from build123d import *

# Parameters (mm, degrees)
SKETCH_1_W          = 159
SKETCH_1_H          = 116
EXTRUDE_1_DEPTH     = 2
SKETCH_3_R          = 1.99
EXTRUDE_3_DEPTH     = 79.5
SKETCH_4_W          = 149
SKETCH_4_H          = 7
CUT_EXTRUDE_2_DEPTH = 79.5
FILLET_3_R          = 2


with BuildPart() as part:
    # 草图1 → 凸台-拉伸1 (new body)
    with BuildSketch(Plane(origin=(0, 0, 0), x_dir=(1, 0, 0), z_dir=(0, 1, 0))):
        Rectangle(SKETCH_1_W, SKETCH_1_H)
    extrude(amount=EXTRUDE_1_DEPTH)

    # 草图3 → 凸台-拉伸3 (add, symmetric)
    # profile 1 of 2: a face of its own
    with BuildSketch(Plane(origin=(0, 0, 0), x_dir=(0, 0, -1), z_dir=(1, 0, 0))):
        with BuildLine():
            Line((-57, 6), (-57, 2))
            Line((-57, 2), (-51, 2))
            Line((-51, 2), (-51, 6))
            ThreePointArc((-51, 6), (-54, 9), (-57, 6))
        make_face()
        with Locations(Location((-54, 6, 0), (0, 0, 180))):
            Circle(SKETCH_3_R, mode=Mode.SUBTRACT)
    # profile 2 of 2: a face of its own
    with BuildSketch(Plane(origin=(0, 0, 0), x_dir=(0, 0, -1), z_dir=(1, 0, 0))):
        with BuildLine():
            Line((51, 2), (51, 6))
            ThreePointArc((51, 6), (54, 9), (57, 6))
            Line((57, 6), (57, 2))
            Line((57, 2), (51, 2))
        make_face()
        with Locations(Location((54, 6, 0), (0, 0, 180))):
            Circle(SKETCH_3_R, mode=Mode.SUBTRACT)
    extrude(amount=EXTRUDE_3_DEPTH, both=True)

    # 草图4 → 切除-拉伸2 (cut, symmetric)
    with BuildSketch(Plane.XY):
        with Locations((0, 5.5)):
            Rectangle(SKETCH_4_W, SKETCH_4_H)
    extrude(amount=CUT_EXTRUDE_2_DEPTH, both=True, mode=Mode.SUBTRACT)

    # 圆角3
    # the kernel refuses this fillet: 2 mm, written as the material it adds along each edge
    with BuildSketch(Plane(origin=(74.5, 2, 57), x_dir=(0, 1, 0), z_dir=(1, 0, 0))) as fillet_3_piece_1:
        with BuildLine():
            CenterArc((1.732050808, 2), FILLET_3_R, 210, 60)
            Line((0, 1), (-0.034641016, 0.98))
            ThreePointArc((-0.034641016, 0.98), (-0.04, 0.5), (-0.04, 0))
            Line((-0.04, 0), (0, -0.04))
            Line((0, -0.04), (1.732050808, -0.04))
            Line((1.732050808, -0.04), (1.732050808, 0))
        make_face()
    extrude(amount=5)
    with BuildSketch(Plane(origin=(74.5, 2, 51), x_dir=(0, 1, 0), z_dir=(1, 0, 0)), Plane(origin=(-79.5, 2, -51), x_dir=(0, 0, 1), z_dir=(1, 0, 0))) as fillet_3_piece_2:
        with BuildLine():
            CenterArc((FILLET_3_R, -FILLET_3_R), FILLET_3_R, 90, 90)
            Line((0, -FILLET_3_R), (-FILLET_3_R * 0.02, -FILLET_3_R))
            Line((-FILLET_3_R * 0.02, -FILLET_3_R), (-FILLET_3_R * 0.02, FILLET_3_R * 0.02))
            Line((-FILLET_3_R * 0.02, FILLET_3_R * 0.02), (FILLET_3_R, FILLET_3_R * 0.02))
            Line((FILLET_3_R, FILLET_3_R * 0.02), (FILLET_3_R, 0))
        make_face()
    extrude(amount=5)
    with BuildSketch(Plane(origin=(74.5, 2, -51), x_dir=(0, 1, 0), z_dir=(1, 0, 0)), Plane(origin=(-79.5, 2, 51), x_dir=(0, 0, -1), z_dir=(1, 0, 0))) as fillet_3_piece_3:
        with BuildLine():
            CenterArc((FILLET_3_R, FILLET_3_R), FILLET_3_R, 180, 90)
            Line((0, FILLET_3_R), (-FILLET_3_R * 0.02, FILLET_3_R))
            Line((-FILLET_3_R * 0.02, FILLET_3_R), (-FILLET_3_R * 0.02, -FILLET_3_R * 0.02))
            Line((-FILLET_3_R * 0.02, -FILLET_3_R * 0.02), (FILLET_3_R, -FILLET_3_R * 0.02))
            Line((FILLET_3_R, -FILLET_3_R * 0.02), (FILLET_3_R, 0))
        make_face()
    extrude(amount=5)
    with BuildSketch(Plane(origin=(74.5, 2, -57), x_dir=(0, 1, 0), z_dir=(1, 0, 0))) as fillet_3_piece_4:
        with BuildLine():
            CenterArc((1.732050808, -2), FILLET_3_R, 90, 60)
            Line((0, -1), (-0.034641016, -0.98))
            ThreePointArc((-0.034641016, -0.98), (-0.04, -0.5), (-0.04, 0))
            Line((-0.04, 0), (0, 0.04))
            Line((0, 0.04), (1.732050808, 0.04))
            Line((1.732050808, 0.04), (1.732050808, 0))
        make_face()
    extrude(amount=5)
    with BuildSketch(Plane(origin=(-79.5, 2, -57), x_dir=(0, 0, -1), z_dir=(1, 0, 0))) as fillet_3_piece_5:
        with BuildLine():
            CenterArc((2, 1.732050808), FILLET_3_R, 180, 60)
            Line((0, 1.732050808), (-0.04, 1.732050808))
            Line((-0.04, 1.732050808), (-0.04, 0))
            Line((-0.04, 0), (0, -0.04))
            ThreePointArc((0, -0.04), (0.5, -0.04), (0.98, -0.034641016))
            Line((0.98, -0.034641016), (1, 0))
        make_face()
    extrude(amount=5)
    with BuildSketch(Plane(origin=(-79.5, 2, 57), x_dir=(0, 0, 1), z_dir=(1, 0, 0))) as fillet_3_piece_6:
        with BuildLine():
            CenterArc((2, -1.732050808), FILLET_3_R, 120, 60)
            Line((0, -1.732050808), (-0.04, -1.732050808))
            Line((-0.04, -1.732050808), (-0.04, 0))
            Line((-0.04, 0), (0, 0.04))
            ThreePointArc((0, 0.04), (0.5, 0.04), (0.98, 0.034641016))
            Line((0.98, 0.034641016), (1, 0))
        make_face()
    extrude(amount=5)


solid = part.part
Here's how the part is built. I have some questions about the finished solid (model axes, mm). A direction names the side the tool comes from. Coordinates: 2 decimals unless noted, no trailing zeros. Order: outer loops, then holes, each group sorted by start corner. A loop starts at its lowest first (then second) coordinate and runs counter-clockwise, first axis right, second up. Notation, with made-up numbers: M 15,-21.75 L 19,-21.75 A19 cw 19,13.25 Z; hole C 40,2.25 d9. An arc over 180 degrees is marked long. Answer as CSV lines item,"result".
Item 1: For pin 1 (2.5 mm diameter, centred on x = -76, y = 5, fed in from +Z); pin 2 (3 mm diameter, centred on x = 3.5, z = -26, fed in from -Y); pin 3 (3.5 mm diameter, centred on y = 6, z = 54, fed in from -X); pin 4 (2 mm diameter, centred on x = -76.5, y = 4.5, fed in from -Z), each with a flat end and sliding along its axis, tell me the tip position at first contact or that it passes through.
Results found:
pin 1,"z = 57"
pin 2,"y = 0"
pin 3,"through"
pin 4,"z = -57.01"
Item 2: Imagine slicing it at A-A on z = -54. Write out the boundary of the cut face in (x, y), plus the area to 3 significant figures.
Results found:
outline,"M -79.5,0 L 79.5,0 L 79.5,4.01 L 74.5,4.01 L 74.5,2 L -74.5,2 L -74.5,4.01 L -79.5,4.01 Z; M -79.5,7.99 L -74.5,7.99 L -74.5,9 L -79.5,9 Z; M 74.5,7.99 L 79.5,7.99 L 79.5,9 L 74.5,9 Z"
area,"348 mm2"
Item 3: Imagine slicing it at B-B on x = 29. Write out the boundary of the cut face in (y, z).
Results found:
outline,"M 0,-58 L 2,-58 L 2,58 L 0,58 Z"
Item 4: Imagine slicing it at C-C on z = -4.5. Write out the boundary of the cut face in (x, y), plus the area to 3 significant figures.
Results found:
outline,"M -79.5,0 L 79.5,0 L 79.5,2 L -79.5,2 Z"
area,"318 mm2"
Item 5: We'd pull the mould along X, two halves only. Please class faces 3 (the face through (-77, 9, 54)), 4 (the face through (79.5, 1, 0)), 5 (the face through (-1, 2, -1)): +X half, -X half, draft (parallel to the pull), parting line (faces both ways), or undercut.
Results found:
face 3,"draft"
face 4,"+X half"
face 5,"undercut"
Item 6: If I drill on line 1 (Z direction, x = -78.35, y = 6); line 2 (Y direction, x = -77.25, z = 54); line 3 (Y direction, x = -27, z = -16), over which ranges is the centre line in solid material (lowest first)?
Results found:
line 1,"-57 to -55.99, -52.01 to -51, 51 to 52.01, 55.99 to 57"
line 2,"0 to 4.01, 7.99 to 9"
line 3,"0 to 2"
Item 7: On a 3-axis mill with a long thin cutter (end or side, diameter ignored), from which of +Z, -Z, +X, -X, +Y, -Y can I reach the whole of each face in a straight line? I mean faces 1 (the face through (77, 9, -54)), 2 (the face through (-74.5, 4, -55)). Say none if no direction works.
Results found:
face 1,"+X, -X, +Y"
face 2,"+Z, -Z, +Y"
